Verification items for this drawing (mm, ordinates from the low corner). A direction names the side the tool comes from. Give positions to 0.01 mm unless a question says otherwise; leave off trailing zeros. Loops run counter-clockwise (first coordinate to the right, second up) from the corner with the lowest first, then second, coordinate; pieces in that order, holes last. Notation, with made-up numbers: (85, 22) -> (103, 22) arc R19 ccw to (103, 50) -> close; hole circle Ø2 at (26, 78.5). An arc over 180 degrees is marked (long way). Write item = value, one per line.
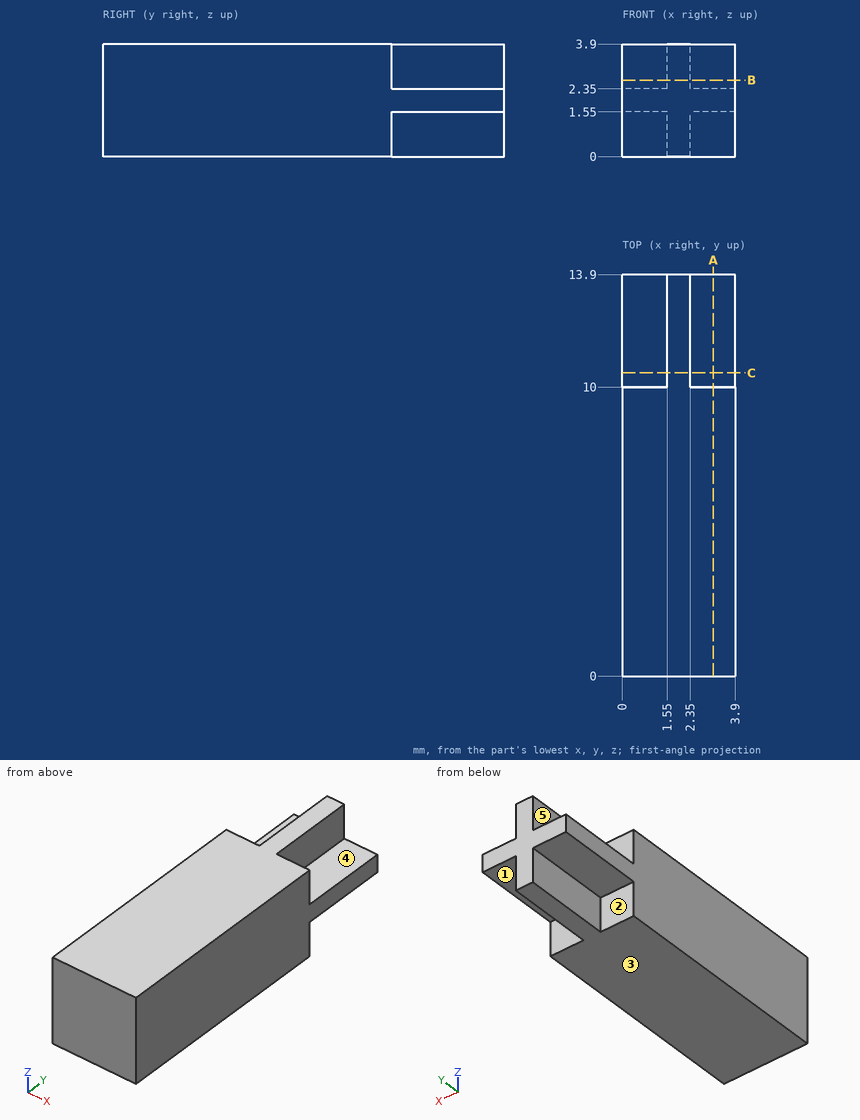
Item 1: Section check A-A, the plane x = 3.15. Record the cut outline in (y, z), plus the area to 3 significant figures.
Answer:
outline = (0, 0) -> (10, 0) -> (10, 1.55) -> (13.9, 1.55) -> (13.9, 2.35) -> (10, 2.35) -> (10, 3.9) -> (0, 3.9) -> close
area = 42.1 mm^2
Item 2: Tool access check on the marked faces 1, 2, 3, 4 and 5. Record the directions out of +Z, -Z, +X, -X, +Y, -Y that give a thin tool (end or side, any length) a straight path to the whole face; none if there is none.
Answer:
face_1 = -Z, +X, +Y
face_2 = -Z, -X, +Y
face_3 = -Z, +X, -X, +Y, -Y
face_4 = +Z, +X, +Y
face_5 = +Z, -X, +Y
Item 3: Thickness scan on L1, parallel to Y at x = 3.2, z = 3.3; L2, parallel to Z at x = 3.4, y = 11.5. Record the ranges inside material, lowest first. Write a range as [from, to].
Answer:
L1 = [0, 10]
L2 = [1.55, 2.35]
Item 4: Section check C-C, the plane y = 10.5. Record the cut outline in (x, z).
Answer:
outline = (0, 1.55) -> (1.55, 1.55) -> (1.55, 0) -> (2.35, 0) -> (2.35, 1.55) -> (3.9, 1.55) -> (3.9, 2.35) -> (2.35, 2.35) -> (2.35, 3.9) -> (1.55, 3.9) -> (1.55, 2.35) -> (0, 2.35) -> close
Item 5: Section check B-B, the plane z = 2.65. Record the cut outline in (x, y), plus the area to 3 significant figures.
Answer:
outline = (0, 0) -> (3.9, 0) -> (3.9, 10) -> (2.35, 10) -> (2.35, 13.9) -> (1.55, 13.9) -> (1.55, 10) -> (0, 10) -> close
area = 42.1 mm^2
Item 6: Gauge pin test, flat ends, axial feed: pin 1 (0.8 mm diameter, centred on x = 3.5, y = 12.5, fed in from +Z); pin 2 (0.8 mm diameter, centred on y = 12, z = 3, fed in from +X); pin 3 (0.8 mm diameter, centred on x = 3.5, z = 1, fed in from +Y). Record the tip position at first contact, or that the pin passes through.
Answer:
pin_1 = 2.35
pin_2 = 2.35
pin_3 = 10
